Work out the finished part from the listing and answer in its coordinate system (mm). A direction names the side the tool comes from. Give positions to 0.01 mm unless a question says otherwise; leave off trailing zeros. Loops run counter-clockwise (first coordinate to the right, second up) from the corner with the lowest first, then second, coordinate; pieces in that order, holes last. Notation, with made-up numbers: M 49,67.5 L 99,67.5 A15 ccw 99,86.5 Z; hole C -28.5,23.25 d9. An arc over 180 degrees is marked long. Answer in a Markdown table with one row per item. Add a question column.
from build123d import *

# Parameters (mm, degrees)
SKETCH1_W           = 230
SKETCH1_H           = 20
BOSS_EXTRUDE1_DEPTH = 7
SKETCH2_R           = 1.75
CUT_EXTRUDE1_DEPTH  = 8
SKETCH3_R           = 5
CUT_EXTRUDE2_DEPTH  = 4


with BuildPart() as part:
    # Sketch1 → Boss-Extrude1 (new body)
    with BuildSketch(Plane.XY):
        Rectangle(SKETCH1_W, SKETCH1_H)
    extrude(amount=BOSS_EXTRUDE1_DEPTH)

    # Sketch2 → Cut-Extrude1 (cut, through all)
    with BuildSketch(Plane.XY.offset(7)):
        with Locations((-100, 0)):
            Circle(SKETCH2_R)
        with Locations((100, 0)):
            Circle(SKETCH2_R)
        with Locations((50, 0)):
            Circle(SKETCH2_R)
        with Locations((-50, 0)):
            Circle(SKETCH2_R)
    extrude(amount=-CUT_EXTRUDE1_DEPTH, mode=Mode.SUBTRACT)

    # Sketch3 → Cut-Extrude2 (cut)
    with BuildSketch(Plane.XY.offset(7)):
        with Locations((-100, 0)):
            Circle(SKETCH3_R)
        with Locations((-50, 0)):
            Circle(SKETCH3_R)
        with Locations((50, 0)):
            Circle(SKETCH3_R)
        with Locations((100, 0)):
            Circle(SKETCH3_R)
    extrude(amount=-CUT_EXTRUDE2_DEPTH, mode=Mode.SUBTRACT)


solid = part.part
(1) Each of these flat-tipped pins is pushed along its axis until it touches: P1, Ø9, axis at x = -50, y = 0, coming from the +Z side; P2, Ø8, axis at x = 100, y = 0, coming from the -Z side. Where does it stop, or does it pass through?
(2) Which of the six approach directions +Z, -Z, +X, -X, +Y, -Y give full straight-line access (tool end or side, diameter ignored) to faces 5 (the face through (-2, 0, 7)), 6 (the face through (45, 0, 5))?
(3) Section A-A, the plane z = 4.5 is taken. Determine the outline of the cut face in (x, y).
(4) The mould has two halves that part along X. Classify faces 1 (the face through (-115, 0, 3)), 2 (the face through (-2, 10, 3)), 3 (the face through (115, 0, 3)), 4 (the face through (-95.381, -1.915, 5.028)): pulls with the +X half, pulls with the -X half, needs draft (parallel to the pull), parting line crosses it, or undercut.
(5) Consider line 1 along X through (y, z) = (0.25, 4.5); line 2 along X through (y, z) = (-2.5, 4); line 3 along Y through (x, z) = (-50, 4.4). Determine where each line is inside the solid, lowest interval first. Write a range as from..to.
Numbers:
| question | item | result |
|---|---|---|
| 1 | P1 | stops at z = 3 |
| 1 | P2 | stops at z = 0 |
| 2 | face 5 | +Z, +X, -X, +Y, -Y |
| 2 | face 6 | +Z |
| 3 | outline | M -115,-10 L 115,-10 L 115,10 L -115,10 Z; hole C -100,0 d10; hole C -50,0 d10; hole C 50,0 d10; hole C 100,0 d10 |
| 4 | face 1 | pulls with the -X half |
| 4 | face 2 | needs draft |
| 4 | face 3 | pulls with the +X half |
| 4 | face 4 | undercut |
| 5 | line 1 | x = -115..-104.99, -95.01..-54.99, -45.01..45.01, 54.99..95.01, 104.99..115 |
| 5 | line 2 | x = -115..-104.33, -95.67..-54.33, -45.67..45.67, 54.33..95.67, 104.33..115 |
| 5 | line 3 | y = -10..-5, 5..10 |
